Source: CAD feature listing. Evaluate the final solid. Frame: model axes, mm. A direction names the side the tool comes from. Give positions to 0.01 mm unless a question says otherwise; leave off trailing zeros. Order: outer loops, then holes, each group sorted by start corner. A loop starts at its lowest first (then second) coordinate and runs counter-clockwise, first axis right, second up.
```python
from build123d import *

# Parameters (mm, degrees)
SKETCH1_R           = 5
BOSS_EXTRUDE1_DEPTH = 5
SKETCH2_R           = 4.9
BOSS_EXTRUDE2_DEPTH = 10
BOSS_EXTRUDE3_START = -1
SKETCH4_R           = 5
BOSS_EXTRUDE3_DEPTH = 1


with BuildPart() as part:
    # Sketch1 → Boss-Extrude1 (new body)
    with BuildSketch(Plane(origin=(0, 0, 0), x_dir=(1, 0, 0), z_dir=(0, 1, 0))):
        with BuildLine():
            Line((0, 0), (15, 0))
            ThreePointArc((15, 0), (22.5, 7.5), (15, 15))
            Line((15, 15), (0, 15))
            ThreePointArc((0, 15), (-7.5, 7.5), (0, 0))
        make_face()
        with Locations(Location((0, 7.5, 0), (0, 0, 270))):
            Circle(SKETCH1_R, mode=Mode.SUBTRACT)
        with Locations(Location((15, 7.5, 0), (0, 0, 270))):
            Circle(SKETCH1_R, mode=Mode.SUBTRACT)
    extrude(amount=BOSS_EXTRUDE1_DEPTH)



with BuildPart() as body_2:
    # Sketch2 → Boss-Extrude2 (new body)
    with BuildSketch(Plane(origin=(0, 5, 0), x_dir=(1, 0, 0), z_dir=(0, 1, 0))):
        with Locations(Location((15, 7.5, 0), (0, 0, 270))):
            Circle(SKETCH2_R)
    extrude(amount=-BOSS_EXTRUDE2_DEPTH)


with BuildPart() as part_1:
    add(part.part)

    add(body_2.part)  # Boss-Extrude3 merges body 2
    # Sketch4 → Boss-Extrude3 (add)
    with BuildSketch(Plane(origin=(0, 5, 0), x_dir=(-1, 0, 0), z_dir=(0, 1, 0)).offset(BOSS_EXTRUDE3_START)):
        with Locations(Location((-15, -7.5, 0), (0, 0, 90))):
            Circle(SKETCH4_R)
    extrude(amount=BOSS_EXTRUDE3_DEPTH)


solid = part_1.part
```
1) Section query A-A, the plane z = -7.5. Return the cut outline in (x, y).
Report:
outline: (-7.5, 0) - (-5, 0) - (-5, 5) - (-7.5, 5) - close; (5, 0) - (10, 0) - (10, 4) - (10.1, 4) - (10.1, -5) - (19.9, -5) - (19.9, 4) - (20, 4) - (20, 0) - (22.5, 0) - (22.5, 5) - (5, 5) - close
2) Material intervals for L1, parallel to Y at x = 13.75, z = -14.5; L2, parallel to Z at x = 18.25, y = -0.25; L3, parallel to Z at x = 16.5, y = -1.5, sorted ascending.
Report:
L1: y = 0 to 5
L2: z = -11.17 to -3.83
L3: z = -12.16 to -2.84
3) Pin query (flat end, axial travel): pin 1 (1.5 mm diameter, centred on y = 4, z = -8.5, fed in from -X); pin 2 (3 mm diameter, centred on x = 7.5, z = -7.5, fed in from -Y); pin 3 (3 mm diameter, centred on y = 1.5, z = -3, fed in from -X). Return the tip coordinate at first contact, or that it passes through.
Report:
pin 1: stops at x = -7.5
pin 2: stops at y = 0
pin 3: stops at x = -6.87
4) Reachability of faces 4 (the flat face through (7, 0, -8)), 5 (the flat face through (7, 2, 0)) from +Z, -Z, +X, -X, +Y, -Y: full face, straight path, thin tool, end or side. Return the list, or none.
Report:
face 4: -Y
face 5: +Z, +X, -X, +Y, -Y
5) Section query B-B, the plane x = 5.75. Return the cut outline in (y, z), and give its area (3 significant figures).
Report:
outline: (0, -15) - (5, -15) - (5, 0) - (0, 0) - close
area: 75.0 mm2
6) Section query D-D, the plane y = -3.5. Return the cut outline in (x, z).
Report:
outline: circle Ø9.8 at (15, -7.5)
7) Draft query along Z for faces 1 (the flat face through (8, 2, -15)), 2 (the cylindrical face through (13.123, -0.437, -2.974)), 3 (the flat face through (15, -5, -8)). Return one class per face: +Z half, -Z half, draft (parallel to the pull), parting line (faces both ways), or undercut.
Report:
face 1: -Z half
face 2: undercut
face 3: draft
8) Section query C-C, the plane z = -5.5. Return the cut outline in (x, y).
Report:
outline: (-7.23, 0) - (-4.58, 0) - (-4.58, 5) - (-7.23, 5) - close; (4.58, 0) - (10.42, 0) - (10.42, 4) - (10.53, 4) - (10.53, -5) - (19.47, -5) - (19.47, 4) - (19.58, 4) - (19.58, 0) - (22.23, 0) - (22.23, 5) - (4.58, 5) - close
